Can you work these out from the model? Positions are in its coordinate system, mm. A direction names the side the tool comes from. Give positions to 0.01 mm unless a question says otherwise; leave off trailing zeros. Order: outer loops, then holes, each group sorted by start corner. A loop starts at its lowest first (then second) coordinate and runs counter-clockwise, first axis right, second up. Notation, with made-up numbers: M 43.5,19.25 L 82.5,19.25 A22 cw 82.5,50.25 Z; hole C -15.75,66.25 d8. An arc over 180 degrees is marked long. Answer as a JSON object with one key per item and string values.
Autodesk Inventor part; units mm, degrees
sketch "Sketch1" plane through (0, 0, 0) normal (0, 0, 1) x (1, 0, 0)
  line L0 (0, 25.4) -> (76.2, 25.4)
  line L1 (76.2, 25.4) -> (76.2, -25.4)
  line L2 (76.2, -25.4) -> (0, -25.4)
  line L3 (0, -25.4) -> (0, 25.4)
  line L4 (-15.24, 0) -> (91.44, 0)
  line L5 (0, 35.56) -> (0, -35.56)
  point P0 (0, 0)
  dimension "d0" = 50.8
  dimension "d1" = 76.2
  dimension "d2" = 25.4
  dimension "d3" = 0
extrude "Extrusion1" add sketch "Sketch1" along normal mid plane 12.7
sketch "Sketch2" plane through (0, 0, 6.35) normal (0, 0, 1) x (1, 0, 0)
  circle A0 centre (50.8, 0) radius 12.7
  line L0 (76.2, -25.4) -> (76.2, 25.4)
  line L1 (0, -25.4) -> (76.2, -25.4)
  point P0 (0, 0)
  dimension "d6" = 25.4
  dimension "d7" = 25.4
  dimension "d8" = 25.4
extrude "Extrusion2" cut sketch "Sketch2" against normal up to surface (12.7 mm away)
sketch "Sketch3" plane through (0, 0, 6.35) normal (0, 0, 1) x (1, 0, 0)
  line L0 (0, -25.4) -> (0, 25.4)
  line L1 (0, -6.35) -> (19.05, -6.35)
  line L2 (19.05, -6.35) -> (19.05, -19.05)
  line L3 (19.05, -19.05) -> (0, -19.05)
  line L4 (0, -25.4) -> (76.2, -25.4)
  point P0 (0, 0)
  dimension "d11" = 12.7
  dimension "d12" = 19.05
  dimension "d13" = 6.35
extrude "Extrusion3" cut sketch "Sketch3" against normal up to surface (12.7 mm away)
chamfer "Chamfer1" distance 12.7 distance2 19.05 1 edges at (76.2, 25.4, 0) measured on face at (76.2, 8.4667, 2.1167)
chamfer "Chamfer2" distance 31.75 distance2 19.05 1 edges at (0, 25.4, 0) measured on face at (19.05, 25.4, 2.1167)
equation "\"d2\" = 0.5 * d0"
properties part number "chap2ex1"
1) I want a section at A-A on y = 0. Write out the boundary of the cut face in (x, z).
Results found:
{"outline": "M 0,-6.35 L 38.1,-6.35 L 38.1,6.35 L 0,6.35 Z; M 63.5,-6.35 L 76.2,-6.35 L 76.2,6.35 L 63.5,6.35 Z"}
2) Thinking about a two-plate mould opening in Y: for faces 1 (the face through (10, -19.05, 0)), 2 (the face through (37.6, 0.4, -6.35)), 3 (the face through (15.65, 15.74, 0.09)), which applies, pulls with the +Y half, pulls with the -Y half, needs draft (parallel to the pull), parting line crosses it, or undercut?
Results found:
{"face 1": "undercut", "face 2": "needs draft", "face 3": "pulls with the +Y half"}
3) I want a section at C-C on z = 5.25. Write out the boundary of the cut face in (x, y).
Results found:
{"outline": "M 0,-25.4 L 76.2,-25.4 L 76.2,12.7 L 57.15,25.4 L 31.75,25.4 L 0,6.35 L 0,-6.35 L 19.05,-6.35 L 19.05,-19.05 L 0,-19.05 Z; hole C 50.8,0 d25.4"}
4) I want a section at B-B on x = 50.8. Write out the boundary of the cut face in (y, z), and give its area (3 significant figures).
Results found:
{"outline": "M -25.4,-6.35 L -12.7,-6.35 L -12.7,6.35 L -25.4,6.35 Z; M 12.7,-6.35 L 25.4,-6.35 L 25.4,6.35 L 12.7,6.35 Z", "area": "323 mm²"}
5) I want a section at D-D on y = -14.5. Write out the boundary of the cut face in (x, z).
Results found:
{"outline": "M 19.05,-6.35 L 76.2,-6.35 L 76.2,6.35 L 19.05,6.35 Z"}
6) I'm going to push flat-ended pins straight in: pin 1 Ø6 at (x, y) = (42, -7.5) entering from +Z; pin 2 Ø1 at (y, z) = (9, -2.5) entering from -X; pin 3 Ø4 at (x, z) = (11.5, -1) entering from +Y. Where does each tip first touch, or does it pass through?
Results found:
{"pin 1": "stops at z = 6.35", "pin 2": "stops at x = 3.58", "pin 3": "stops at y = 14.45"}
7) For faces 4 (the face through (9, -6.35, 0)), 5 (the face through (37.6, 0.4, 6.35)), which set-ups out of +Z, -Z, +X, -X, +Y, -Y let a thin tool reach every point of the face, with its end or its side?
Results found:
{"face 4": "+Z, -Z, -X", "face 5": "+Z, +X, -X, +Y, -Y"}
8) I need wall thicknesses on L1, parallel to Y at x = 50.8, z = -0.25; L2, parallel to X at y = -13, z = 4.25; L3, parallel to X at y = 7.5, z = -1.75. Which ranges of each line are inside material? Lowest first, please.
Results found:
{"L1": "y = -25.4 to -12.7, 12.7 to 25.4", "L2": "x = 19.05 to 76.2", "L3": "x = 1.92 to 40.55, 61.05 to 76.2"}
